Input: part model. Units: mm. Frame: model coordinates. A direction names the side the tool comes from. Coordinates: 2 decimals unless noted, no trailing zeros. Order: outer loops, then holes, each group sorted by start corner. A loop starts at its lowest first (then second) coordinate and runs counter-clockwise, first axis right, second up. Notation, with made-up numbers: M 29,62.5 L 76,62.5 A21 ccw 76,101.5 Z; hole C 17.5,21.25 d11. An arc over 180 degrees is marked long. One line per item, written item: value.
```python
from build123d import *

# Parameters (mm, degrees)
BOSS_EXTRUDE1_DEPTH = 1
BOSS_EXTRUDE2_START = 1
BOSS_EXTRUDE2_DEPTH = 1
CUT_EXTRUDE1_DEPTH  = 10


with BuildPart() as part:
    # Sketch1 → Boss-Extrude1 (new body)
    with BuildSketch(Plane.XY):
        with BuildLine():
            Line((3384.198156919, -60.590855349), (3421.54984535, -71.809205111))
            ThreePointArc((3421.54984535, -71.809205111), (3422.311317421, -71.732090109), (3422.795230945, -71.139119504))
            Line((3422.795230945, -71.139119504), (3432.575330737, -38.576109077))
            ThreePointArc((3432.575330737, -38.576109077), (3432.498215735, -37.814637007), (3431.90524513, -37.330723482))
            Line((3431.90524513, -37.330723482), (3394.553556699, -26.112373721))
            ThreePointArc((3394.553556699, -26.112373721), (3393.792084629, -26.189488722), (3393.308171105, -26.782459328))
            Line((3393.308171105, -26.782459328), (3383.528071313, -59.345469754))
            ThreePointArc((3383.528071313, -59.345469754), (3383.605186314, -60.106941825), (3384.198156919, -60.590855349))
        make_face()
    extrude(amount=-BOSS_EXTRUDE1_DEPTH)

    # Sketch1_4 → Boss-Extrude2 (add)
    # profile 1 of 2: a face of its own
    with BuildSketch(Plane.XY.offset(BOSS_EXTRUDE2_START)):
        with BuildLine():
            Line((3424.710702146, -71.714419492), (3434.490801939, -39.151409065))
            ThreePointArc((3434.490801939, -39.151409065), (3434.259456934, -36.866992853), (3432.480545118, -35.415252281))
            Line((3432.480545118, -35.415252281), (3395.128856687, -24.196902519))
            ThreePointArc((3395.128856687, -24.196902519), (3392.844440476, -24.428247524), (3391.392699903, -26.20715934))
            Line((3391.392699903, -26.20715934), (3381.612600111, -58.770169767))
            ThreePointArc((3381.612600111, -58.770169767), (3381.843945116, -61.054585978), (3383.622856932, -62.506326551))
            Line((3383.622856932, -62.506326551), (3420.974545362, -73.724676312))
            ThreePointArc((3420.974545362, -73.724676312), (3423.258961574, -73.493331308), (3424.710702146, -71.714419492))
        make_face()
        with BuildLine():
            ThreePointArc((3421.54984535, -71.809205111), (3422.311317421, -71.732090109), (3422.795230945, -71.139119504))
            Line((3422.795230945, -71.139119504), (3432.575330737, -38.576109077))
            ThreePointArc((3432.575330737, -38.576109077), (3432.498215735, -37.814637007), (3431.90524513, -37.330723482))
            Line((3431.90524513, -37.330723482), (3394.553556699, -26.112373721))
            ThreePointArc((3394.553556699, -26.112373721), (3393.792084629, -26.189488722), (3393.308171105, -26.782459328))
            Line((3393.308171105, -26.782459328), (3383.528071313, -59.345469754))
            ThreePointArc((3383.528071313, -59.345469754), (3383.605186314, -60.106941825), (3384.198156919, -60.590855349))
            Line((3384.198156919, -60.590855349), (3421.54984535, -71.809205111))
        make_face(mode=Mode.SUBTRACT)
    # profile 2 of 2: a face of its own
    with BuildSketch(Plane.XY.offset(BOSS_EXTRUDE2_START)):
        with BuildLine():
            Line((3384.198156919, -60.590855349), (3421.54984535, -71.809205111))
            ThreePointArc((3421.54984535, -71.809205111), (3422.311317421, -71.732090109), (3422.795230945, -71.139119504))
            Line((3422.795230945, -71.139119504), (3432.575330737, -38.576109077))
            ThreePointArc((3432.575330737, -38.576109077), (3432.498215735, -37.814637007), (3431.90524513, -37.330723482))
            Line((3431.90524513, -37.330723482), (3394.553556699, -26.112373721))
            ThreePointArc((3394.553556699, -26.112373721), (3393.792084629, -26.189488722), (3393.308171105, -26.782459328))
            Line((3393.308171105, -26.782459328), (3383.528071313, -59.345469754))
            ThreePointArc((3383.528071313, -59.345469754), (3383.605186314, -60.106941825), (3384.198156919, -60.590855349))
        make_face()
    extrude(amount=-BOSS_EXTRUDE2_DEPTH)

    # Sketch2 → Cut-Extrude1 (cut)
    with BuildSketch(Plane(origin=(0, 0, -1), x_dir=(-1, 0, 0), z_dir=(0, 0, -1))):
        Polygon((-3455.741612738, -34.933179244), (-3387.643444689, -14.48031354), (-3380.69590789, -37.612256774), (-3448.79407594, -58.065122478), align=None)
    extrude(amount=-CUT_EXTRUDE1_DEPTH, mode=Mode.SUBTRACT)


solid = part.part
```
(1) Ray query, line 1 (Z direction, x = 3384.5, y = -52.5); line 2 (Y direction, x = 3398, z = 0.25); line 3 (Y direction, x = 3404, z = -0.25). Return the intervals inside material, ascending. Write a range as from..to.
Data:
line 1: z = 0..1
line 2: y = -66.82..-42.81
line 3: y = -66.54..-44.61
(2) Cut plane C-C on x = 3427. Output: boundary loops of the cut face in (y, z), plus the area to 3 significant figures.
Data:
outline: M -64.09,0 L -57.14,0 L -57.14,-1 L -51.52,-1 L -51.52,1 L -64.09,1 Z
area: 18.2 mm2
(3) Access query for faces 1 (the flat face through (3404, -67, 0)), 2 (the cylindrical face through (3383.6, -60.1, -0.5)), 3 (the flat face through (3402.61, -66.12, -0.49)). Directions: +Z, -Z, +X, -X, +Y, -Y. A direction counts if a zero-diameter tool reaches every point of the face in a straight line with its end or side. Return the directions, or none.
Data:
face 1: -Z
face 2: -Z, -X
face 3: -Z, -X, -Y
(4) Cut plane B-B on y = -67.5. Output: boundary loops of the cut face in (x, z), plus the area to 3 significant figures.
Data:
outline: M 3400.25,0 L 3407.2,0 L 3407.2,-1 L 3423.89,-1 L 3423.89,0 L 3425.98,0 L 3425.98,1 L 3400.25,1 Z
area: 42.4 mm2
(5) First-contact query: pin 1 (1 mm diameter, centred on x = 3391, y = -66.5, fed in from +Z). Flat tip, straight axial feed; report the tip coordinate or a pass-through.
Data:
pin 1: passes through
(6) Cut plane A-A on z = 0.5. Output: boundary loops of the cut face in (x, y).
Data:
outline: M 3381.61,-58.77 A3 ccw 3383.62,-62.51 L 3420.97,-73.72 A3 ccw 3424.71,-71.71 L 3430.46,-52.56 L 3387.37,-39.62 Z
(7) Cut plane D-D on y = -63. Output: boundary loops of the cut face in (x, z).
Data:
outline: M 3385.27,0 L 3392.22,0 L 3392.22,-1 L 3425.24,-1 L 3425.24,0 L 3427.33,0 L 3427.33,1 L 3385.27,1 Z
